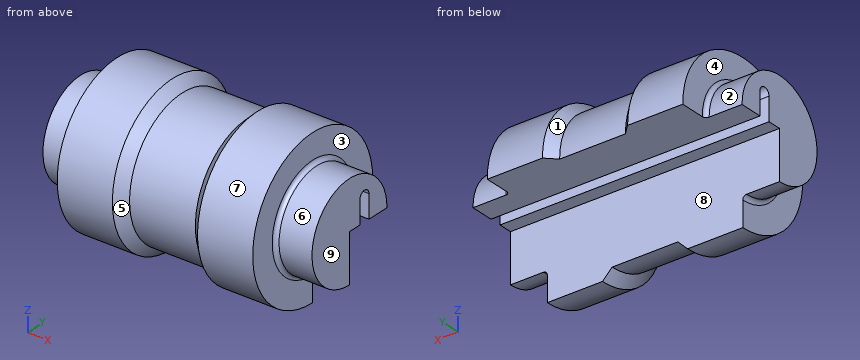
```python
from build123d import *

# Parameters (mm, degrees)
REVOLVE2_ANGLE     = 270
CUT_EXTRUDE1_DEPTH = 151.069983674


with BuildPart() as part:
    # Sketch1 → Revolve2 (revolve)
    with BuildSketch(Plane.XY):
        with BuildLine():
            Line((0, 0), (139, 0))
            Line((139, 0), (139, 25))
            Line((139, 25), (122, 25))
            ThreePointArc((122, 25), (120.585786438, 25.585786438), (120, 27))
            Line((120, 27), (120, 40))
            Line((120, 40), (91.5, 40))
            Line((91.5, 40), (86.5, 35))
            Line((86.5, 35), (52.5, 35))
            Line((52.5, 35), (47.5, 40))
            Line((47.5, 40), (19, 40))
            Line((19, 40), (19, 27))
            ThreePointArc((19, 27), (18.414213562, 25.585786438), (17, 25))
            Line((17, 25), (0, 25))
            Line((0, 25), (0, 0))
        make_face()
    revolve(axis=Axis((0, 0, 0), (1, 0, 0)), revolution_arc=REVOLVE2_ANGLE)

    # Sketch2 → Cut-Extrude1 (cut, through all)
    with BuildSketch(Plane(origin=(139, 0, 0), x_dir=(0, 0, -1), z_dir=(1, 0, 0))):
        with BuildLine():
            Line((0, 7), (-12, 7))
            ThreePointArc((-12, 7), (-15, 10), (-12, 13))
            Line((-12, 13), (0, 13))
            Line((0, 13), (0, 7))
        make_face()
    extrude(amount=-CUT_EXTRUDE1_DEPTH, mode=Mode.SUBTRACT)


solid = part.part
```
Part model, mm, in its own coordinate system. Face numbers are marked on the shaded views. A direction names the side the tool comes from. Round coordinates to 2 decimals unless told otherwise and drop trailing zeros. Write each loop counter-clockwise with the first axis right and the second up, starting at its lowest first coordinate (ties: lowest second). Pieces come first, ordered by that corner, then holes. Notation, with made-up numbers: M 23,74.5 L 39,74.5 A31 ccw 39,99.5 Z; hole C 24,-26.75 d9. An arc over 180 degrees is marked long. Answer as CSV lines item,"result". Start each with the question number.
1) Drop flat-ended pins along their axis: pin 1 (1 mm diameter, centred on x = 24, z = 16, fed in from +Y); pin 2 (8 mm diameter, centred on x = 94.5, y = -29.5, fed in from -Z); pin 3 (5 mm diameter, centred on x = 17, z = -13.5, fed in from -Y). Give the stop position or say it passes through.
2) Drill centre lines: L1, parallel to X at y = -14.5, z = -32; L2, parallel to Z at x = 81.5, y = -1.5; L3, parallel to X at y = -29, z = -23. Where is each one in solid material? Low to high.
3) Band-saw the part on A-A (x = 89). List the corners of the cut face in (y, z).
4) Mould opens along X. For the marked faces 1, 2, 3 and 4 say: +X half, -X half, draft (parallel to the pull), parting line (faces both ways), or undercut.
5) Band-saw the part on B-B (x = 112). List the corners of the cut face in (y, z), then the cut area to 3 significant figures.
6) Which spindle directions (+Z, -Z, +X, -X, +Y, -Y) get a long thin tool onto all of the face, cutting with end or side? Do the marked faces 5, 6, 7, 8 and 9. Say none if no direction does.
Worked out:
1,pin 1,"y = 36.87"
1,pin 2,"z = -30.82"
1,pin 3,"y = -38.16"
2,L1,"19 to 52.37, 86.63 to 120"
2,L2,"-34.97 to 34.97"
2,L3,"19 to 50.49, 88.51 to 120"
3,outline,"M 0,-37.5 L 0,0 L 7,0 L 7,12 A3 cw 13,12 L 13,0 L 37.5,0 A37.5 ccw long Z"
4,face 1,"undercut"
4,face 2,"draft"
4,face 3,"+X half"
4,face 4,"-X half"
5,outline,"M 0,-40 L 0,0 L 7,0 L 7,12 A3 cw 13,12 L 13,0 L 40,0 A40 ccw long Z"
5,area,"3,680 mm²"
6,face 5,"none"
6,face 6,"+X"
6,face 7,"+X, -X"
6,face 8,"-Z, +X, -X, +Y"
6,face 9,"+Z, -Z, +X, +Y, -Y"
